```python
from build123d import *
from build123d.topology import SkipClean

# Parameters (mm, degrees)
SKETCH1_R           = 100
BOSS_EXTRUDE2_DEPTH = 1120
SKETCH4_R           = 37.5
CUT_EXTRUDE1_DEPTH  = 1100
SKETCH6_R           = 30.030042901
CUT_EXTRUDE2_DEPTH  = 1129.893263334
SKETCH7_R           = 5
CUT_EXTRUDE3_DEPTH  = 1200
FILLET1_R           = 25
SKETCH8_W           = 276.180333513
SKETCH8_H           = 316.248560879
CUT_EXTRUDE4_DEPTH  = 65
SKETCH9_R           = 7.5
CUT_EXTRUDE5_DEPTH  = 2
BOSS_EXTRUDE3_START = 223.21458
BOSS_EXTRUDE3_DEPTH = 223.21458
SKETCH11_R          = 125
BOSS_EXTRUDE4_DEPTH = 10
SKETCH12_W          = 75
SKETCH12_H          = 223.21458
CUT_EXTRUDE6_DEPTH  = 123
CUT_EXTRUDE7_REACH  = 1292.381
SKETCH13_R          = 10


with BuildPart() as part:
    # Sketch1 → Boss-Extrude2 (new body)
    with BuildSketch(Plane(origin=(0, 0, 0), x_dir=(1, 0, 0), z_dir=(0, 1, 0))):
        with Locations(Location((0, 0, 0), (0, 0, 270))):
            Circle(SKETCH1_R)
    extrude(amount=BOSS_EXTRUDE2_DEPTH)

    # Sketch4 → Cut-Extrude1 (cut)
    with BuildSketch(Plane(origin=(0, 1120, 0), x_dir=(1, 0, 0), z_dir=(0, 1, 0))):
        with Locations(Location((55, 0, 0), (0, 0, 270))):
            Circle(SKETCH4_R)
        with Locations(Location((0, 55, 0), (0, 0, 270))):
            Circle(SKETCH4_R)
        with Locations(Location((-55, 0, 0), (0, 0, 270))):
            Circle(SKETCH4_R)
        with Locations(Location((0, -55, 0), (0, 0, 270))):
            Circle(SKETCH4_R)
    extrude(amount=-CUT_EXTRUDE1_DEPTH, mode=Mode.SUBTRACT)

    # Sketch6 → Cut-Extrude2 (cut, through all)
    with BuildSketch(Plane(origin=(0, 1120, 0), x_dir=(1, 0, 0), z_dir=(0, 1, 0))):
        with Locations((-70.710678119, 70.710678119)):
            Circle(SKETCH6_R)
        with Locations((70.710678119, 70.710678119)):
            Circle(SKETCH6_R)
        with Locations((70.710678119, -70.710678119)):
            Circle(SKETCH6_R)
        with Locations((-70.710678119, -70.710678119)):
            Circle(SKETCH6_R)
    extrude(amount=-CUT_EXTRUDE2_DEPTH, mode=Mode.SUBTRACT)

    # Sketch7 → Cut-Extrude3 (cut)
    with BuildSketch(Plane(origin=(0, 1120, 0), x_dir=(1, 0, 0), z_dir=(0, 1, 0))):
        with Locations(Location((0, 0, 0), (0, 0, 270))):
            Circle(SKETCH7_R)
    extrude(amount=-CUT_EXTRUDE3_DEPTH, mode=Mode.SUBTRACT)

    # Fillet1
    fillet1_edges = [part.edges().sort_by_distance(p)[0] for p in [
        (-46.528605162, 560, 88.51603754),
        (-88.51603754, 560, 46.528605162),
        (88.51603754, 560, 46.528605162),
        (46.528605162, 560, 88.51603754),
        (46.528605162, 560, -88.51603754),
        (88.51603754, 560, -46.528605162),
        (-88.51603754, 560, -46.528605162),
        (-46.528605162, 560, -88.51603754),
    ]]
    fillet(fillet1_edges, radius=FILLET1_R)

    # Sketch8 → Cut-Extrude4 (cut)
    with BuildSketch(Plane(origin=(0, 1120, 0), x_dir=(1, 0, 0), z_dir=(0, 1, 0))):
        with Locations((9.785456368, -2.918303702)):
            Rectangle(SKETCH8_W, SKETCH8_H)
    extrude(amount=-CUT_EXTRUDE4_DEPTH, mode=Mode.SUBTRACT)

    # Sketch9 → Cut-Extrude5 (cut)
    with BuildSketch(Plane(origin=(0, 1055, 0), x_dir=(1, 0, 0), z_dir=(0, 1, 0))):
        with Locations(Location((0, 0, 0), (0, 0, 270))):
            Circle(SKETCH9_R)
    extrude(amount=-CUT_EXTRUDE5_DEPTH, mode=Mode.SUBTRACT)

    # Sketch10 → Boss-Extrude3 (add)
    with SkipClean():  # the faces are left unmerged after this step: merging them gives an invalid solid
        with BuildSketch(Plane.XZ.offset(BOSS_EXTRUDE3_START)):
            with BuildLine():
                ThreePointArc((20.990620884, 97.772152656), (0, 100), (-20.990620884, 97.772152656))
                ThreePointArc((-20.990620884, 97.772152656), (-35.556079582, 88.575114519), (-40.71464911, 72.139565913))
                ThreePointArc((-40.71464911, 72.139565913), (-49.476231144, 49.476231144), (-72.139565913, 40.71464911))
                ThreePointArc((-72.139565913, 40.71464911), (-88.575114519, 35.556079582), (-97.772152656, 20.990620884))
                ThreePointArc((-97.772152656, 20.990620884), (-100, 0), (-97.772152656, -20.990620884))
                ThreePointArc((-97.772152656, -20.990620884), (-88.575114519, -35.556079582), (-72.139565913, -40.71464911))
                ThreePointArc((-72.139565913, -40.71464911), (-49.476231144, -49.476231144), (-40.71464911, -72.139565913))
                ThreePointArc((-40.71464911, -72.139565913), (-35.556079582, -88.575114519), (-20.990620884, -97.772152656))
                ThreePointArc((-20.990620884, -97.772152656), (0, -100), (20.990620884, -97.772152656))
                ThreePointArc((20.990620884, -97.772152656), (35.556079582, -88.575114519), (40.71464911, -72.139565913))
                ThreePointArc((40.71464911, -72.139565913), (49.476231144, -49.476231144), (72.139565913, -40.71464911))
                ThreePointArc((72.139565913, -40.71464911), (88.575114519, -35.556079582), (97.772152656, -20.990620884))
                ThreePointArc((97.772152656, -20.990620884), (100, 0), (97.772152656, 20.990620884))
                ThreePointArc((97.772152656, 20.990620884), (88.575114519, 35.556079582), (72.139565913, 40.71464911))
                ThreePointArc((72.139565913, 40.71464911), (49.476231144, 49.476231144), (40.71464911, 72.139565913))
                ThreePointArc((40.71464911, 72.139565913), (35.556079582, 88.575114519), (20.990620884, 97.772152656))
            make_face()
        extrude(amount=-BOSS_EXTRUDE3_DEPTH)

    # Sketch11 → Boss-Extrude4 (add)
    with SkipClean():  # the faces are left unmerged after this step: merging them gives an invalid solid
        with BuildSketch(Plane.XZ.offset(223.21458)):
            with Locations(Location((0, 0, 0), (0, 0, 270))):
                Circle(SKETCH11_R)
        extrude(amount=-BOSS_EXTRUDE4_DEPTH)

    # Sketch12 → Cut-Extrude6 (cut, symmetric)
    with SkipClean():  # the faces are left unmerged after this step: merging them gives an invalid solid
        with BuildSketch(Plane(origin=(0, 0, 0), x_dir=(0, 0, -1), z_dir=(1, 0, 0))):
            with Locations((0, -101.60729)):
                Rectangle(SKETCH12_W, SKETCH12_H)
        extrude(amount=CUT_EXTRUDE6_DEPTH, both=True, mode=Mode.SUBTRACT)

    # Sketch13 → Cut-Extrude7 (cut, up to next)
    with BuildSketch(Plane.XZ.offset(223.21458), mode=Mode.PRIVATE) as cut_extrude7_sk1:
        with Locations(Location((65, 65, 0), (0, 0, 270))):
            Circle(SKETCH13_R)
    cut_extrude7_tool1 = extrude(cut_extrude7_sk1.sketch, amount=-CUT_EXTRUDE7_REACH, mode=Mode.PRIVATE) & part.part
    # Sketch13 → Cut-Extrude7 (cut, up to next)
    with BuildSketch(Plane.XZ.offset(223.21458), mode=Mode.PRIVATE) as cut_extrude7_sk2:
        with Locations(Location((65, -65, 0), (0, 0, 270))):
            Circle(SKETCH13_R)
    cut_extrude7_tool2 = extrude(cut_extrude7_sk2.sketch, amount=-CUT_EXTRUDE7_REACH, mode=Mode.PRIVATE) & part.part
    # Sketch13 → Cut-Extrude7 (cut, up to next)
    with BuildSketch(Plane.XZ.offset(223.21458), mode=Mode.PRIVATE) as cut_extrude7_sk3:
        with Locations(Location((-65, -65, 0), (0, 0, 270))):
            Circle(SKETCH13_R)
    cut_extrude7_tool3 = extrude(cut_extrude7_sk3.sketch, amount=-CUT_EXTRUDE7_REACH, mode=Mode.PRIVATE) & part.part
    # Sketch13 → Cut-Extrude7 (cut, up to next)
    with BuildSketch(Plane.XZ.offset(223.21458), mode=Mode.PRIVATE) as cut_extrude7_sk4:
        with Locations(Location((-65, 65, 0), (0, 0, 270))):
            Circle(SKETCH13_R)
    cut_extrude7_tool4 = extrude(cut_extrude7_sk4.sketch, amount=-CUT_EXTRUDE7_REACH, mode=Mode.PRIVATE) & part.part
    add(cut_extrude7_tool1.solids().sort_by_distance((65, -223.21458, 65))[0], mode=Mode.SUBTRACT)
    add(cut_extrude7_tool2.solids().sort_by_distance((65, -223.21458, -65))[0], mode=Mode.SUBTRACT)
    add(cut_extrude7_tool3.solids().sort_by_distance((-65, -223.21458, -65))[0], mode=Mode.SUBTRACT)
    add(cut_extrude7_tool4.solids().sort_by_distance((-65, -223.21458, 65))[0], mode=Mode.SUBTRACT)


solid = part.part
```
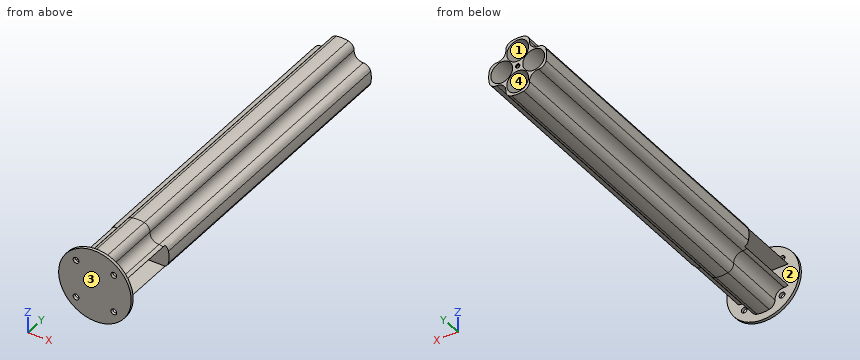
Part model, mm, in its own coordinate system. Face numbers are marked on the shaded views. A direction names the side the tool comes from. Round coordinates to 2 decimals unless told otherwise and drop trailing zeros. Loops run counter-clockwise (first coordinate to the right, second up) from the corner with the lowest first, then second, coordinate; pieces in that order, holes last. Notation, with made-up numbers: (53, 15.5) -> (74, 15.5) arc R28 ccw to (74, 34.5) -> close; hole circle Ø10 at (56.5, 40). An arc over 180 degrees is marked (long way). Use CSV: the item, a comma, the result in double quotes. Start each with the question number.
1) Wall check: L1, parallel to X at y = 608.5, z = 0; L2, parallel to Y at x = 6.5, z = -2; L3, parallel to Y at x = 89, z = 17. Give the ranges that are in metal, low to high. Write a range as [from, to].
2) Drop flat-ended pins along their axis: P1, Ø18, axis at x = 65, z = 65, coming from the -Y side; P2, Ø9, axis at x = 0, z = 0, coming from the +Y side; P3, Ø1.5, axis at x = -63, y = 722, coming from the +Z side; P4, Ø10, axis at y = 669, z = -55, coming from the -X side. Give the stop position or say it passes through.
3) Which spindle directions (+Z, -Z, +X, -X, +Y, -Y) get a long thin tool onto all of the face, cutting with end or side? Do the marked faces 1 and 2. Say none if no direction does.
4) Cut at B-B, the plane y = 117. Give the number of separate pieces and of enclosed holes in the cut face, plus the area to 3 significant figures.
5) Pull direction Z, two halves, no side cores. Call the marked faces 3 and 4: +Z half, -Z half, draft (parallel to the pull), parting line (faces both ways), or undercut.
6) Cut at A-A, the plane y = -105. Write the cut outline in (x, z).
Determined:
1,L1,"x = [-100, -92.5], [-17.5, -5], [5, 17.5], [92.5, 100]"
1,L2,"y = [-223.21, -213.21], [10, 1053]"
1,L3,"y = [-223.21, -213.21], [10, 1055]"
2,P1,"passes through"
2,P2,"stops at y = -213.21"
2,P3,"stops at z = 41.9"
2,P4,"stops at x = -48.97"
3,face 1,"+Y"
3,face 2,"none"
4,separate pieces,"1"
4,enclosed holes,"5"
4,area,"7,510 mm2"
5,face 3,"draft"
5,face 4,"undercut"
6,outline,"(-85.64, -37.5) arc R25 ccw to (-72.14, -40.71) arc R30.03 cw to (-40.71, -72.14) arc R25 ccw to (-20.99, -97.77) arc R100 ccw to (20.99, -97.77) arc R25 ccw to (40.71, -72.14) arc R30.03 cw to (72.14, -40.71) arc R25 ccw to (85.64, -37.5) -> close; (-85.64, 37.5) -> (85.64, 37.5) arc R25 ccw to (72.14, 40.71) arc R30.03 cw to (40.71, 72.14) arc R25 ccw to (20.99, 97.77) arc R100 ccw to (-20.99, 97.77) arc R25 ccw to (-40.71, 72.14) arc R30.03 cw to (-72.14, 40.71) arc R25 ccw to start"
